Answer from the drawing. Dimensions are ordinates in mm from the lowest x, y and z of the part. Round coordinates to 2 decimals unless told otherwise and drop trailing zeros. Order: outer loops, then holes, each group sorted by start corner. A loop starts at its lowest first (then second) coordinate and runs counter-clockwise, first axis right, second up. Notation, with made-up numbers: (-36, 39.25) -> (10, 39.25) arc R16 ccw to (10, 49.25) -> close; hole circle Ø2 at (12, 48). An arc over 180 degrees is marked (long way). Use a Markdown table: item, result. Add a question column.
1. Section A-A, the plane z = 5.5 is taken. Give the number of separate pieces and of enclosed holes in the cut face, then the cut area to 3 significant figures.
2. Consider L1, parallel to Y at x = 1.45, z = 5.5; L2, parallel to Z at x = 5.5, y = 30.5; L3, parallel to Y at x = 2.75, z = 1.25. Determine where each line is inside the solid, lowest interval first. Write a range as [from, to].
3. Section C-C, the plane y = 10.5 is taken. Give the vertices of the cut face in (x, z).
4. The mould has two halves that part along X. Classify the marked faces 1 and 2: +X half, -X half, draft (parallel to the pull), parting line (faces both ways), or undercut.
5. Section D-D, the plane z = 3.25 is taken. Give the vertices of the cut face in (x, y).
6. Section B-B, the plane x = 5.5 is taken. Give the vertices of the cut face in (y, z), then the cut area to 3 significant figures.
7. Given pin 1 (5 mm diameter, centred on y = 29.5, z = 4, fed in from +X); pin 2 (2 mm diameter, centred on x = 9, y = 24.5, fed in from -Z); pin 3 (4 mm diameter, centred on x = 7.5, y = 16.5, fed in from -Z), each flat-ended and moving along its own axis, determine where each tip first touches the part or whether it passes through.
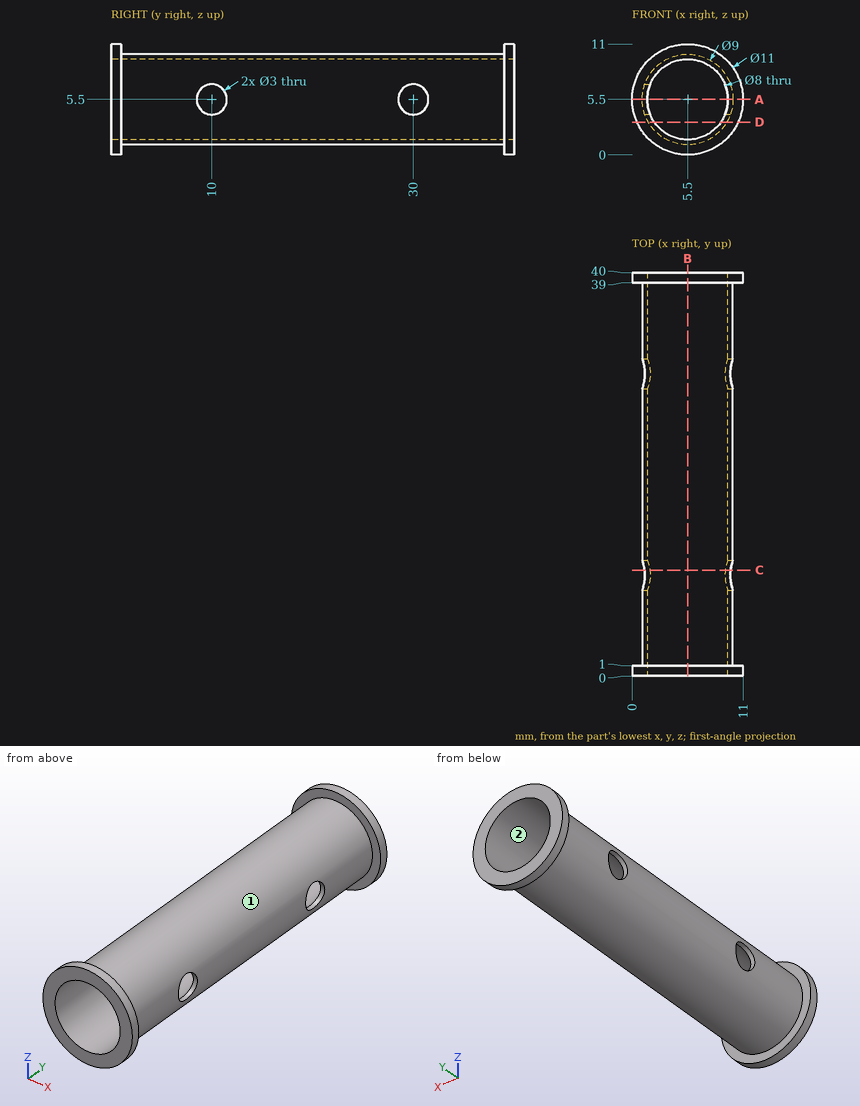
Verdict:
| question | item | result |
|---|---|---|
| 1 | separate pieces | 6 |
| 1 | enclosed holes | 0 |
| 1 | area | 38.0 mm2 |
| 2 | L1 | y = [0, 8.5], [11.5, 28.5], [31.5, 40] |
| 2 | L2 | z = [1, 1.5], [9.5, 10] |
| 2 | L3 | y = [0, 1], [39, 40] |
| 3 | outline | (1.23, 4.09) arc R4.5 ccw to (9.77, 4.09) -> (9.24, 4.09) arc R4 cw to (1.76, 4.09) -> close; (1.23, 6.91) -> (1.76, 6.91) arc R4 cw to (9.24, 6.91) -> (9.77, 6.91) arc R4.5 ccw to start |
| 4 | face 1 | parting line |
| 4 | face 2 | undercut |
| 5 | outline | (0.48, 0) -> (2.19, 0) -> (2.19, 40) -> (0.48, 40) -> (0.48, 39) -> (1.6, 39) -> (1.6, 1) -> (0.48, 1) -> close; (8.81, 0) -> (10.52, 0) -> (10.52, 1) -> (9.4, 1) -> (9.4, 39) -> (10.52, 39) -> (10.52, 40) -> (8.81, 40) -> close |
| 6 | outline | (0, 0) -> (1, 0) -> (1, 1) -> (39, 1) -> (39, 0) -> (40, 0) -> (40, 1.5) -> (0, 1.5) -> close; (0, 9.5) -> (40, 9.5) -> (40, 11) -> (39, 11) -> (39, 10) -> (1, 10) -> (1, 11) -> (0, 11) -> close |
| 6 | area | 44.0 mm2 |
| 7 | pin 1 | stops at x = 10 |
| 7 | pin 2 | stops at z = 1.76 |
| 7 | pin 3 | stops at z = 1 |
